For this review, take the finished solid that the model builds, in its own axes (mm). Face numbers are marked on the shaded views. A direction names the side the tool comes from. Coordinates: 2 decimals unless noted, no trailing zeros. Order: outer loops, then holes, each group sorted by start corner. A loop starts at its lowest first (then second) coordinate and runs counter-clockwise, first axis right, second up.
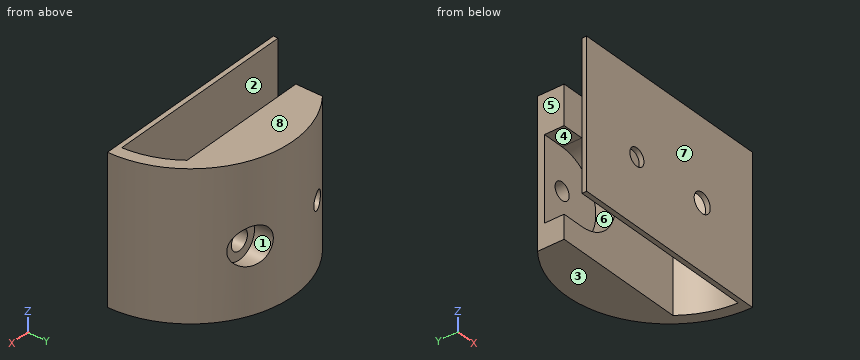
from build123d import *

# Parameters (mm, degrees)
PAD009_DEPTH      = 16
PAD009_DEPTH_BACK = 7.5
POCKET_DEPTH      = 8
HOLE_D            = 3.2
HOLE_DEPTH        = 25
HOLE_CBORE_D      = 6
HOLE_CBORE_DEPTH  = 3.4
SKETCH045_R       = 1.4
POCKET016_DEPTH   = 16


with BuildPart() as part:
    # Sketch → Pad009 (new body, two sides)
    with BuildSketch(Plane.XY) as pad009_sk:
        with BuildLine():
            Line((-16.5, 0), (16.5, 0))
            ThreePointArc((16.5, 0), (7.3229092579, 14.7859730826), (-10, 13.1244047484))
            Line((-10, 8.85), (-10, 13.1244047484))
            Line((11.6433725784, 8.85), (-10, 8.85))
            ThreePointArc((14.6057565706, 0.75), (13.7352355375, 5.0233385044), (11.6433725784, 8.85))
            Line((-16.4829457319, 0.75), (14.6057565706, 0.75))
            ThreePointArc((-16.4829457319, 0.75), (-16.495735882, 0.3750969368), (-16.5, 0))
        make_face()
    extrude(amount=PAD009_DEPTH)
    extrude(pad009_sk.sketch, amount=-PAD009_DEPTH_BACK)

    # Sketch033 (on DatumPlane) → Pocket (cut)
    with BuildSketch(Plane.ZX.offset(12)):
        with BuildLine():
            Line((9.707631, -19.5547157413), (-3.707631, -19.5547157413))
            Line((-3.707631, -19.5547157413), (-3.707631, -6.5))
            ThreePointArc((9.707631, -6.5), (3, 0.207631), (-3.707631, -6.5))
            Line((9.707631, -6.5), (9.707631, -19.5547157413))
        make_face()
    extrude(amount=-POCKET_DEPTH, mode=Mode.SUBTRACT)

    # Hole
    with Locations(Plane(origin=(0, 16.5, 0), x_dir=(1, 0, 0), z_dir=(0, 1, 0))):
        with Locations((6.5, -3)):
            CounterBoreHole(HOLE_D / 2, HOLE_CBORE_D / 2, HOLE_CBORE_DEPTH, depth=HOLE_DEPTH)

    # Sketch045 → Pocket016 (cut)
    with BuildSketch(Plane.XZ):
        with Locations((-6.5, 3)):
            Circle(SKETCH045_R)
    extrude(amount=-POCKET016_DEPTH, mode=Mode.SUBTRACT)


solid = part.part
1. Take a section at C-C, the plane x = 10.5. Give the boundary of the cut face in (y, z), plus the area to 3 significant figures.
Answer below:
outline: (0, -7.5) - (0.75, -7.5) - (0.75, 16) - (0, 16) - close; (8.85, -7.5) - (12.73, -7.5) - (12.73, 16) - (8.85, 16) - close
area: 109 mm2
2. Take a section at B-B, the plane y = 9.25. Give the boundary of the cut face in (x, z).
Answer below:
outline: (-10, -7.5) - (13.66, -7.5) - (13.66, 16) - (-10, 16) - (-10, 9.71) - (-6.5, 9.71) arc R6.71 cw to (-6.5, -3.71) - (-10, -3.71) - close; hole circle Ø3.2 at (6.5, 3)
3. The part is to be moulded in two halves that separate along Y. For the marked faces 6, 7 and 8, say which applies: +Y half, -Y half, draft (parallel to the pull), parting line (faces both ways), or undercut.
Answer below:
face 6: undercut
face 7: -Y half
face 8: draft
4. Clearance check with flat-ended pins moving along their axes: pin 1 Ø1.7 at (x, z) = (-6.5, 3) entering from -Y; pin 2 Ø3.5 at (y, z) = (12, 1.5) entering from -X; pin 3 Ø5 at (x, z) = (6.5, 3) entering from +Y; pin 4 Ø1.5 at (x, z) = (-7, -4.5) entering from +Y. State where each tip first meets the part, or that it passes through.
Answer below:
pin 1: passes through
pin 2: stops at x = -10
pin 3: stops at y = 13.1
pin 4: stops at y = 15.27
5. Take a section at D-D, the plane z = 3. Give the number of separate pieces and of enclosed holes in the cut face, plus the area to 3 significant figures.
Answer below:
separate pieces: 5
enclosed holes: 0
area: 111 mm2
6. To check wall thickness, follow L1, parallel to Z at x = 6.5, y = 0.5; L2, parallel to Y at x = 3.5, z = 6.25; L3, parallel to Z at x = -6.5, y = 13.7. State the ranges of each line that lie inside material, in increasing order.
Answer below:
L1: z = -7.5 to 1.4, 4.6 to 16
L2: y = 0 to 0.75, 8.85 to 16.12
L3: z = -7.5 to 1.6, 4.4 to 16
7. Machinability: for the marked faces 1, 2, 3, 4 and 5, which of the approach directions +Z, -Z, +X, -X, +Y, -Y give a long, thin tool a straight path to every point of the face, cutting with its end or side? Answer none if there is none.
Answer below:
face 1: +Y
face 2: +Z, -Z, -X
face 3: -Z, +X, -X, +Y, -Y
face 4: -X
face 5: +Z, -Z, -X, +Y
8. Take a section at A-A, the plane x = 5.5. Give the boundary of the cut face in (y, z), plus the area to 3 significant figures.
Answer below:
outline: (0, -7.5) - (0.75, -7.5) - (0.75, 1.75) - (0, 1.75) - close; (0, 4.25) - (0.75, 4.25) - (0.75, 16) - (0, 16) - close; (8.85, -7.5) - (15.56, -7.5) - (15.56, 0.17) - (13.1, 0.17) - (13.1, 1.75) - (8.85, 1.75) - close; (8.85, 4.25) - (13.1, 4.25) - (13.1, 5.83) - (15.56, 5.83) - (15.56, 16) - (8.85, 16) - close
area: 149 mm2
